Build history of the part. All positions in model axes, mm. A direction names the side the tool comes from. Give positions to 0.01 mm unless a question says otherwise; leave off trailing zeros. Loops run counter-clockwise (first coordinate to the right, second up) from the corner with the lowest first, then second, coordinate; pieces in that order, holes last. Notation, with made-up numbers: (20.25, 85) - (67.25, 85) arc R32 ccw to (67.25, 118) - close; hole circle Ø5 at (31, -2). An arc over 180 degrees is marked (long way). Return JSON: item names as keys, results as strings. Group by question number.
1) Slice it at A-A (x = -244). List the corners of the cut face in (y, z), and give its area (3 significant figures).
2) Mould opens along Z. For faces 1 (the face through (-245, 20, -45)), 2 (the face through (-199, 100, -45)) say: released by +Z, released by -Z, zero draft, split by the parting line, or undercut.
3) Slice it at B-B (z = -46.25). List the corners of the cut face in (x, y), and give its area (3 significant figures).
4) 3-axis set-ups, long thin cutter, end or side, ignore diameter. For faces 3 (the face through (-155, 50, -42.5)), 4 (the face through (-199, 0, -45)), 5 (the face through (-245, 78, -47.5)): which of +Z, -Z, +X, -X, +Y, -Y reach the whole face in a straight line?
Autodesk Inventor part; units mm, degrees
ref_plane "YZ Plane" through (0, 0, 0) normal (1, 0, 0) x (0, 1, 0)
ref_plane "XZ Plane" through (0, 0, 0) normal (0, 1, 0) x (-1, 0, 0)
ref_plane "XY Plane" through (0, 0, 0) normal (0, 0, 1) x (1, 0, 0)
sketch "Sketch1" plane through (0, 0, 0) normal (0, 1, 0) x (-1, 0, 0)
  line L0 (400, -50) -> (400, 50)
  line L1 (400, 50) -> (390, 50)
  line L2 (390, 50) -> (390, -40)
  line L3 (390, -40) -> (300, -40)
  line L4 (300, -40) -> (300, -50)
  line L5 (300, -50) -> (400, -50)
  line L6 (250, -50) -> (250, -40)
  line L7 (250, -40) -> (150, -40)
  line L8 (150, -40) -> (150, -50)
  line L9 (150, -50) -> (250, -50)
  line L10 (100, -50) -> (100, -40)
  line L11 (100, -40) -> (10, -40)
  line L12 (10, -40) -> (10, 50)
  line L13 (10, 50) -> (0, 50)
  line L14 (0, 50) -> (0, -50)
  line L15 (0, -50) -> (100, -50)
  point P0 (0, 0)
  dimension "d0" = 100
  dimension "d1" = 100
  dimension "d2" = 10
  dimension "d3" = 10
  dimension "d4" = 100
  dimension "d5" = 100
  dimension "d6" = 100
  dimension "d7" = 10
  dimension "d8" = 10
  dimension "d9" = 50
  dimension "d10" = 50
  dimension "d11" = 400
  dimension "d12" = 50
  dimension "d13" = 50
extrude "Extrusion1" add sketch "Sketch1" along normal blind 100
sketch "Sketch2" plane through (0, 0, 0) normal (1, 0, 0) x (0, 1, 0)
  point P0 (0, 0)
sketch "Sketch3" plane through (0, 0, 50) normal (1, 0, 0) x (0, 0, -1)
  line L0 (92.5, 80) -> (97.5, 80)
  line L1 (97.5, 80) -> (97.5, 75)
  line L2 (97.5, 75) -> (92.5, 75)
  line L3 (92.5, 75) -> (92.5, 80)
  line L4 (97.5, 20) -> (92.5, 20)
  line L5 (92.5, 20) -> (92.5, 25)
  line L6 (92.5, 25) -> (97.5, 25)
  line L7 (97.5, 25) -> (97.5, 20)
  line L8 (0, 100) -> (100, 100)
  line L9 (100, 0) -> (100, 100)
  line L10 (0, 0) -> (100, 0)
  line L11 (92.5, 52.5) -> (97.5, 52.5)
  line L12 (97.5, 52.5) -> (97.5, 47.5)
  line L13 (97.5, 47.5) -> (92.5, 47.5)
  line L14 (92.5, 47.5) -> (92.5, 52.5)
  point P0 (50, 0)
  dimension "d16" = 20
  dimension "d17" = 5
  dimension "d18" = 5
  dimension "d19" = 2.5
  dimension "d20" = 20
  dimension "d21" = 5
  dimension "d22" = 5
  dimension "d24" = 7.5
  dimension "d25" = 5
  dimension "d26" = 5
  dimension "d27" = 2.5
  dimension "d28" = 22.5
extrude "Extrusion2" cut sketch "Sketch3" against normal blind 320
sketch "Sketch4" plane through (0, 0, 50) normal (1, 0, 0) x (0, 0, -1)
  line L0 (97.5, 75) -> (92.5, 75)
  line L1 (97.5, 80) -> (97.5, 75)
  line L2 (92.5, 80) -> (97.5, 80)
  line L3 (92.5, 75) -> (92.5, 80)
  line L4 (97.5, 47.5) -> (92.5, 47.5)
  line L5 (97.5, 52.5) -> (97.5, 47.5)
  line L6 (92.5, 52.5) -> (97.5, 52.5)
  line L7 (92.5, 47.5) -> (92.5, 52.5)
  line L8 (92.5, 25) -> (97.5, 25)
  line L9 (92.5, 20) -> (92.5, 25)
  line L10 (97.5, 20) -> (92.5, 20)
  line L11 (97.5, 25) -> (97.5, 20)
  line L12 (92.5, 80) -> (97.5, 80)
  line L13 (97.5, 80) -> (97.5, 75)
  line L14 (97.5, 75) -> (92.5, 75)
  line L15 (92.5, 75) -> (92.5, 80)
  line L16 (92.5, 52.5) -> (97.5, 52.5)
  line L17 (97.5, 52.5) -> (97.5, 47.5)
  line L18 (97.5, 47.5) -> (92.5, 47.5)
  line L19 (92.5, 47.5) -> (92.5, 52.5)
  line L20 (92.5, 25) -> (97.5, 25)
  line L21 (97.5, 25) -> (97.5, 20)
  line L22 (97.5, 20) -> (92.5, 20)
  line L23 (92.5, 20) -> (92.5, 25)
  point P0 (50, 0)
extrude "Extrusion3" add sketch "Sketch4" against normal blind 80
sketch "Sketch6" plane through (-250, 0, -40) normal (0, 0, 1) x (1, 0, 0)
  line L0 (-50, 80) -> (-50, 75)
  line L1 (-50, 80) -> (-70, 80)
  line L2 (-70, 80) -> (-70, 75)
  line L3 (-50, 75) -> (-70, 75)
  line L4 (-50, 52.5) -> (-50, 47.5)
  line L5 (-50, 52.5) -> (-70, 52.5)
  line L6 (-70, 52.5) -> (-70, 47.5)
  line L7 (-50, 47.5) -> (-70, 47.5)
  line L8 (-50, 25) -> (-50, 20)
  line L9 (-50, 25) -> (-70, 25)
  line L10 (-70, 25) -> (-70, 20)
  line L11 (-50, 20) -> (-70, 20)
  line L12 (0, 75) -> (0, 80)
  line L13 (100, 75) -> (0, 75)
  line L14 (100, 80) -> (100, 75)
  line L15 (100, 80) -> (0, 80)
  line L16 (0, 47.5) -> (0, 52.5)
  line L17 (100, 47.5) -> (0, 47.5)
  line L18 (100, 52.5) -> (100, 47.5)
  line L19 (100, 52.5) -> (0, 52.5)
  line L20 (0, 20) -> (0, 25)
  line L21 (100, 20) -> (0, 20)
  line L22 (100, 25) -> (100, 20)
  line L23 (100, 25) -> (0, 25)
  line L24 (170, 75) -> (170, 80)
  line L25 (170, 80) -> (150, 80)
  line L26 (150, 75) -> (150, 80)
  line L27 (170, 75) -> (150, 75)
  line L28 (170, 47.5) -> (170, 52.5)
  line L29 (170, 52.5) -> (150, 52.5)
  line L30 (150, 47.5) -> (150, 52.5)
  line L31 (170, 47.5) -> (150, 47.5)
  line L32 (170, 20) -> (170, 25)
  line L33 (170, 25) -> (150, 25)
  line L34 (150, 20) -> (150, 25)
  line L35 (170, 20) -> (150, 20)
  line L36 (-70, 80) -> (-60, 80)
  line L37 (-60, 80) -> (-60, 20)
  line L38 (-60, 20) -> (-70, 20)
  line L39 (-70, 20) -> (-70, 80)
  line L40 (10, 80) -> (90, 80)
  line L41 (90, 80) -> (90, 20)
  line L42 (90, 20) -> (10, 20)
  line L43 (10, 20) -> (10, 80)
  line L44 (160, 80) -> (170, 80)
  line L45 (170, 80) -> (170, 20)
  line L46 (170, 20) -> (160, 20)
  line L47 (160, 20) -> (160, 80)
  line L48 (0, 0) -> (0, 100)
  line L49 (100, 0) -> (100, 100)
  line L50 (10, 25) -> (90, 25)
  line L51 (90, 25) -> (90, 20)
  line L52 (90, 20) -> (10, 20)
  line L53 (10, 20) -> (10, 25)
  point P0 (250, 0)
  point P1 (160, 25)
  point P2 (160, 20)
  point P3 (160, 52.5)
  point P4 (160, 47.5)
  point P5 (160, 75)
  point P6 (10, 75)
  point P7 (90, 75)
  point P8 (90, 80)
  point P9 (10, 52.5)
  point P10 (10, 47.5)
  point P11 (90, 47.5)
  point P12 (90, 52.5)
  point P13 (10, 25)
  point P14 (10, 20)
  point P15 (-60, 25)
  point P16 (-60, 47.5)
  point P17 (-60, 52.5)
  point P18 (-60, 75)
  point P19 (90, 25)
  point P20 (90, 25)
  dimension "d33" = 10
  dimension "d34" = 10
extrude "Extrusion4" add sketch "Sketch6" against normal blind 10 contours L37 L3 L2 L1 | L37 L5 L39 L3 | L37 L7 L6 L5 | L37 L9 L39 L7 | L37 L11 L10 L9 | L43 L15 L41 L13 | L19 L41 L17 L43 | L23 L41 L21 L43 | L27 L47 L25 L24 | L45 L29 L47 L27 | L28 L31 L47 L29 | L45 L33 L47 L31 | L32 L35 L47 L33
sketch "Sketch8" plane through (0, 100, 0) normal (0, 1, 0) x (1, 0, 0)
  line L0 (-300, 50) -> (-400, 50)
  line L1 (-400, 50) -> (-400, -50)
  line L2 (0, 50) -> (-100, 50)
  line L3 (0, -50) -> (0, 50)
  line L4 (-400, 50) -> (-300, 50)
  line L5 (-300, 50) -> (-300, -50)
  line L6 (-300, -50) -> (-400, -50)
  line L7 (-400, -50) -> (-400, 50)
  line L8 (0, 50) -> (-100, 50)
  line L9 (-100, 50) -> (-100, -50)
  line L10 (-100, -50) -> (0, -50)
  line L11 (0, -50) -> (0, 50)
  point P0 (0, 0)
  dimension "d44" = 100
  dimension "d45" = 100
  dimension "d46" = 100
extrude "Extrusion6" cut sketch "Sketch8" against normal through all
properties part number "Soccer Goal Split"
Results:
{
 "1": {"outline": "(0, -50) - (100, -50) - (100, -40) - (0, -40) - close; hole (20, -47.5) - (25, -47.5) - (25, -42.5) - (20, -42.5) - close; hole (47.5, -47.5) - (52.5, -47.5) - (52.5, -42.5) - (47.5, -42.5) - close; hole (75, -47.5) - (80, -47.5) - (80, -42.5) - (75, -42.5) - close", "area": "925 mm2"},
 "2": {"face 1": "undercut", "face 2": "zero draft"},
 "3": {"outline": "(-250, 0) - (-150, 0) - (-150, 20) - (-160, 20) - (-160, 25) - (-150, 25) - (-150, 47.5) - (-160, 47.5) - (-160, 52.5) - (-150, 52.5) - (-150, 75) - (-160, 75) - (-160, 80) - (-150, 80) - (-150, 100) - (-250, 100) - (-250, 80) - (-240, 80) - (-240, 75) - (-250, 75) - (-250, 52.5) - (-240, 52.5) - (-240, 47.5) - (-250, 47.5) - (-250, 25) - (-240, 25) - (-240, 20) - (-250, 20) - close", "area": "9,700 mm2"},
 "4": {"face 3": "+X", "face 4": "+Z, -Z, +X, -X, -Y", "face 5": "-X"}
}
